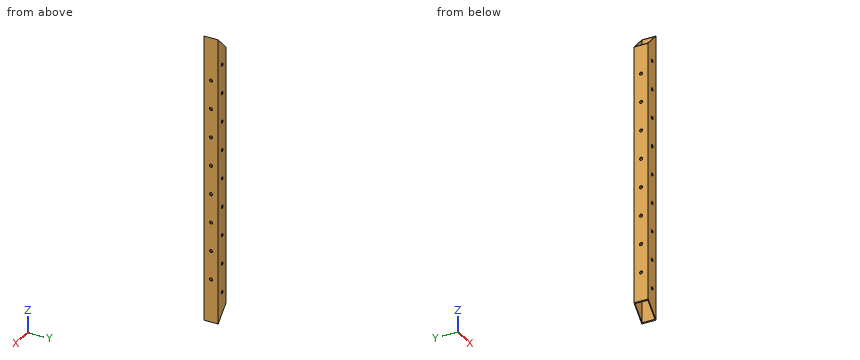
from build123d import *

# Parameters (mm, degrees)
SKETCH_1_R          = 2.2
EXTRUDE_1_DEPTH     = 5
CUT_EXTRUDE_2_DEPTH = 5
SKETCH_3_W          = 20
SKETCH_3_H          = 15
EXTRUDE_2_DEPTH     = 400
SKETCH_4_W          = 18
SKETCH_4_H          = 18
CUT_EXTRUDE_4_DEPTH = 400
CUT_EXTRUDE_5_DEPTH = 400
CUT_EXTRUDE_START   = -400
SKETCH_6_R          = 2.2
CUT_EXTRUDE_6_DEPTH = 400
SKETCH_7_R          = 2.2
CUT_EXTRUDE_7_DEPTH = 40


with BuildPart() as part:
    # 草图1 → 凸台-拉伸1 (new body)
    with BuildSketch(Plane(origin=(0, 0, 0), x_dir=(1, 0, 0), z_dir=(0, 1, 0))):
        Polygon((40, 200), (80, 200), (80, 205), (120, 205), (120, 200), (160, 200), (160, 205), (200, 205), (205, 205), (205, 200), (205, 160), (200, 160), (200, 120), (205, 120), (205, 80), (200, 80), (200, 40), (205, 40), (205, -40), (200, -40), (200, -80), (205, -80), (205, -120), (200, -120), (200, -160), (205, -160), (205, -200), (205, -205), (200, -205), (160, -205), (160, -200), (120, -200), (120, -205), (80, -205), (80, -200), (40, -200), (40, -205), (-40, -205), (-40, -200), (-80, -200), (-80, -205), (-120, -205), (-120, -200), (-160, -200), (-160, -205), (-200, -205), (-205, -205), (-205, -200), (-205, -160), (-200, -160), (-200, -120), (-205, -120), (-205, -80), (-200, -80), (-200, -40), (-205, -40), (-205, 40), (-200, 40), (-200, 80), (-205, 80), (-205, 120), (-200, 120), (-200, 160), (-205, 160), (-205, 200), (-205, 205), (-200, 205), (-160, 205), (-160, 200), (-120, 200), (-120, 205), (-80, 205), (-80, 200), (-40, 200), (-40, 205), (40, 205), align=None)
        with Locations(Location((-190, 0, 0), (0, 0, 270))):
            Circle(SKETCH_1_R, mode=Mode.SUBTRACT)
        with Locations(Location((-190, 40, 0), (0, 0, 270))):
            Circle(SKETCH_1_R, mode=Mode.SUBTRACT)
        with Locations(Location((-190, 80, 0), (0, 0, 270))):
            Circle(SKETCH_1_R, mode=Mode.SUBTRACT)
        with Locations(Location((-190, 120, 0), (0, 0, 270))):
            Circle(SKETCH_1_R, mode=Mode.SUBTRACT)
        with Locations(Location((-190, 160, 0), (0, 0, 270))):
            Circle(SKETCH_1_R, mode=Mode.SUBTRACT)
        with Locations(Location((-190, -160, 0), (0, 0, 270))):
            Circle(SKETCH_1_R, mode=Mode.SUBTRACT)
        with Locations(Location((-190, -120, 0), (0, 0, 270))):
            Circle(SKETCH_1_R, mode=Mode.SUBTRACT)
        with Locations(Location((-190, -80, 0), (0, 0, 270))):
            Circle(SKETCH_1_R, mode=Mode.SUBTRACT)
        with Locations(Location((-190, -40, 0), (0, 0, 270))):
            Circle(SKETCH_1_R, mode=Mode.SUBTRACT)
        with Locations(Location((0, 190, 0), (0, 0, 270))):
            Circle(SKETCH_1_R, mode=Mode.SUBTRACT)
        with Locations(Location((40, 190, 0), (0, 0, 270))):
            Circle(SKETCH_1_R, mode=Mode.SUBTRACT)
        with Locations(Location((80, 190, 0), (0, 0, 270))):
            Circle(SKETCH_1_R, mode=Mode.SUBTRACT)
        with Locations(Location((120, 190, 0), (0, 0, 270))):
            Circle(SKETCH_1_R, mode=Mode.SUBTRACT)
        with Locations(Location((160, 190, 0), (0, 0, 270))):
            Circle(SKETCH_1_R, mode=Mode.SUBTRACT)
        with Locations(Location((-160, 190, 0), (0, 0, 270))):
            Circle(SKETCH_1_R, mode=Mode.SUBTRACT)
        with Locations(Location((-120, 190, 0), (0, 0, 270))):
            Circle(SKETCH_1_R, mode=Mode.SUBTRACT)
        with Locations(Location((-80, 190, 0), (0, 0, 270))):
            Circle(SKETCH_1_R, mode=Mode.SUBTRACT)
        with Locations(Location((-40, 190, 0), (0, 0, 270))):
            Circle(SKETCH_1_R, mode=Mode.SUBTRACT)
        with Locations(Location((190, 0, 0), (0, 0, 270))):
            Circle(SKETCH_1_R, mode=Mode.SUBTRACT)
        with Locations(Location((190, -40, 0), (0, 0, 270))):
            Circle(SKETCH_1_R, mode=Mode.SUBTRACT)
        with Locations(Location((190, -80, 0), (0, 0, 270))):
            Circle(SKETCH_1_R, mode=Mode.SUBTRACT)
        with Locations(Location((190, -120, 0), (0, 0, 270))):
            Circle(SKETCH_1_R, mode=Mode.SUBTRACT)
        with Locations(Location((190, -160, 0), (0, 0, 270))):
            Circle(SKETCH_1_R, mode=Mode.SUBTRACT)
        with Locations(Location((190, 160, 0), (0, 0, 270))):
            Circle(SKETCH_1_R, mode=Mode.SUBTRACT)
        with Locations(Location((190, 120, 0), (0, 0, 270))):
            Circle(SKETCH_1_R, mode=Mode.SUBTRACT)
        with Locations(Location((190, 80, 0), (0, 0, 270))):
            Circle(SKETCH_1_R, mode=Mode.SUBTRACT)
        with Locations(Location((190, 40, 0), (0, 0, 270))):
            Circle(SKETCH_1_R, mode=Mode.SUBTRACT)
        with Locations(Location((0, -190, 0), (0, 0, 270))):
            Circle(SKETCH_1_R, mode=Mode.SUBTRACT)
        with Locations(Location((-40, -190, 0), (0, 0, 270))):
            Circle(SKETCH_1_R, mode=Mode.SUBTRACT)
        with Locations(Location((-80, -190, 0), (0, 0, 270))):
            Circle(SKETCH_1_R, mode=Mode.SUBTRACT)
        with Locations(Location((-120, -190, 0), (0, 0, 270))):
            Circle(SKETCH_1_R, mode=Mode.SUBTRACT)
        with Locations(Location((-160, -190, 0), (0, 0, 270))):
            Circle(SKETCH_1_R, mode=Mode.SUBTRACT)
        with Locations(Location((160, -190, 0), (0, 0, 270))):
            Circle(SKETCH_1_R, mode=Mode.SUBTRACT)
        with Locations(Location((120, -190, 0), (0, 0, 270))):
            Circle(SKETCH_1_R, mode=Mode.SUBTRACT)
        with Locations(Location((80, -190, 0), (0, 0, 270))):
            Circle(SKETCH_1_R, mode=Mode.SUBTRACT)
        with Locations(Location((40, -190, 0), (0, 0, 270))):
            Circle(SKETCH_1_R, mode=Mode.SUBTRACT)
    extrude(amount=EXTRUDE_1_DEPTH)

    # 草图2 → 切除-拉伸2 (cut)
    with BuildSketch(Plane(origin=(0, 5, 0), x_dir=(1, 0, 0), z_dir=(0, 1, 0))):
        Polygon((-262.338764773, 278.332609162), (-269.219830918, -271.432403188), (296.387975763, -278.51176372), (303.269041909, 271.25324863), align=None)
        Polygon((-180, -180), (-180, -200), (-200, -200), (-200, -160), (-200, 200), (-180, 200), (-180, 180), (-180, -160), align=None, mode=Mode.SUBTRACT)
    extrude(amount=-CUT_EXTRUDE_2_DEPTH, mode=Mode.SUBTRACT)

    # 草图3 → 凸台-拉伸2 (add)
    with BuildSketch(Plane.XY.offset(200)):
        with Locations((-190, -7.5)):
            Rectangle(SKETCH_3_W, SKETCH_3_H)
    extrude(amount=-EXTRUDE_2_DEPTH)

    # 草图4 → 切除-拉伸4 (cut)
    with BuildSketch(Plane.XY.offset(200)):
        with Locations((-190, -5)):
            Rectangle(SKETCH_4_W, SKETCH_4_H)
    extrude(amount=-CUT_EXTRUDE_4_DEPTH, mode=Mode.SUBTRACT)

    # 草图5 → 切除-拉伸5 (cut)
    with BuildSketch(Plane(origin=(0, 5, 0), x_dir=(1, 0, 0), z_dir=(0, 1, 0))):
        Polygon((-180, -200), (-200, -180), (-200, -200), align=None)
        Polygon((-200, 200), (-180, 200), (-200, 180), align=None)
    extrude(amount=-CUT_EXTRUDE_5_DEPTH, mode=Mode.SUBTRACT)

    # 草图6 → 切除-拉伸6 (cut)
    with BuildSketch(Plane(origin=(0, 5, 0), x_dir=(1, 0, 0), z_dir=(0, 1, 0)).offset(CUT_EXTRUDE_START)):
        with Locations(Location((-190, 160, 0), (0, 0, 90))):
            Circle(SKETCH_6_R)
        with Locations(Location((-190, 120, 0), (0, 0, 90))):
            Circle(SKETCH_6_R)
        with Locations(Location((-190, 80, 0), (0, 0, 90))):
            Circle(SKETCH_6_R)
        with Locations(Location((-190, 40, 0), (0, 0, 90))):
            Circle(SKETCH_6_R)
        with Locations(Location((-190, 0, 0), (0, 0, 90))):
            Circle(SKETCH_6_R)
        with Locations(Location((-190, -40, 0), (0, 0, 90))):
            Circle(SKETCH_6_R)
        with Locations(Location((-190, -80, 0), (0, 0, 90))):
            Circle(SKETCH_6_R)
        with Locations(Location((-190, -120, 0), (0, 0, 90))):
            Circle(SKETCH_6_R)
        with Locations(Location((-190, -160, 0), (0, 0, 90))):
            Circle(SKETCH_6_R)
    extrude(amount=CUT_EXTRUDE_6_DEPTH, mode=Mode.SUBTRACT)

    # 草图7 → 切除-拉伸7 (cut)
    with BuildSketch(Plane.ZY.offset(200)):
        with Locations((-140, -5)):
            Circle(SKETCH_7_R)
        with Locations((-100, -5)):
            Circle(SKETCH_7_R)
        with Locations((-60, -5)):
            Circle(SKETCH_7_R)
        with Locations((-20, -5)):
            Circle(SKETCH_7_R)
        with Locations((20, -5)):
            Circle(SKETCH_7_R)
        with Locations((60, -5)):
            Circle(SKETCH_7_R)
        with Locations((100, -5)):
            Circle(SKETCH_7_R)
        with Locations((140, -5)):
            Circle(SKETCH_7_R)
    extrude(amount=-CUT_EXTRUDE_7_DEPTH, mode=Mode.SUBTRACT)


solid = part.part
For this review, take the finished solid that the model builds, in its own axes (mm). Give positions to 0.01 mm unless a question says otherwise; leave off trailing zeros. Order: outer loops, then holes, each group sorted by start corner. A loop starts at its lowest first (then second) coordinate and runs counter-clockwise, first axis right, second up. Notation, with made-up numbers: M -21,18 L -14,18 A5 ccw -14,23 Z; hole C 36,62.25 d5. An arc over 180 degrees is marked long. Answer in a Markdown table with one row per item. Add a question column.
(1) Consider section A-A on y = 0.5. State the section outline as (x, z) points.
(2) For pin 1 (2.5 mm diameter, centred on x = -190, z = 40, fed in from +Y), flat-tipped, find the tip position at first contact; note if it passes through.
(3) Wall thickness on probe 1 along Y at (x, z) = (-188, -168); probe 2 along X at (y, z) = (-13, -115); probe 3 along X at (y, z) = (-14.5, -80): over which ranges is each line inside the solid? List them lowest first. Write a range as [from, to].
Evaluation:
| question | item | result |
|---|---|---|
| 1 | outline | M -200,-180 L -199,-181 L -199,181 L -200,180 Z; M -181,-199 L -180,-200 L -180,200 L -181,199 Z |
| 2 | pin 1 | passes through |
| 3 | probe 1 | y = [-15, -14], [4, 5] |
| 3 | probe 2 | x = [-200, -199], [-181, -180] |
| 3 | probe 3 | x = [-200, -192.2], [-187.8, -180] |
